from build123d import *

# Parameters (mm, degrees)
SKETCH_1_W          = 170
SKETCH_1_H          = 106
EXTRUDE_1_DEPTH     = 14
SKETCH_2_R          = 2
CUT_EXTRUDE_1_DEPTH = 5
SKETCH_3_W          = 154
SKETCH_3_H          = 87
CUT_EXTRUDE_2_DEPTH = 1


with BuildPart() as part:
    # 草图1 → 凸台-拉伸1 (new body)
    with BuildSketch(Plane.XY):
        Rectangle(SKETCH_1_W, SKETCH_1_H)
    extrude(amount=-EXTRUDE_1_DEPTH)

    # 草图2 → 切除-拉伸1 (cut)
    with BuildSketch(Plane(origin=(0, 0, -14), x_dir=(-1, 0, 0), z_dir=(0, 0, -1))):
        with Locations((37.5, 37.5)):
            Circle(SKETCH_2_R)
        with Locations((-37.5, 37.5)):
            Circle(SKETCH_2_R)
        with Locations((-37.5, -37.5)):
            Circle(SKETCH_2_R)
        with Locations((37.5, -37.5)):
            Circle(SKETCH_2_R)
    extrude(amount=-CUT_EXTRUDE_1_DEPTH, mode=Mode.SUBTRACT)

    # 草图3 → 切除-拉伸2 (cut)
    with BuildSketch(Plane.XY):
        with Locations((0, 1.5)):
            Rectangle(SKETCH_3_W, SKETCH_3_H)
    extrude(amount=-CUT_EXTRUDE_2_DEPTH, mode=Mode.SUBTRACT)


solid = part.part
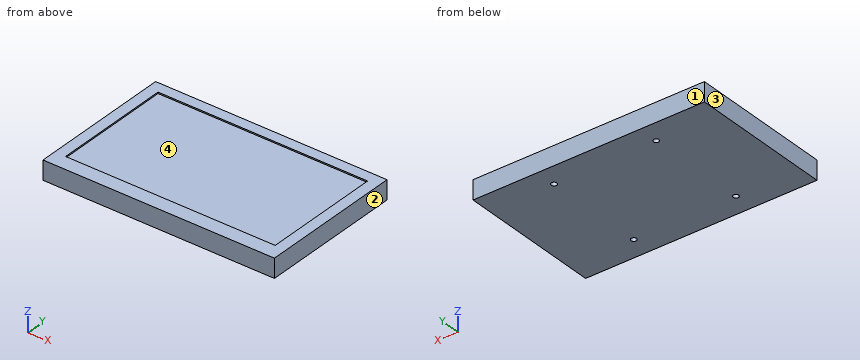
Design review of the part built by this model. Coordinates are the model's own, in mm. Face numbers are marked on the shaded views. Give positions to 0.01 mm unless a question says otherwise; leave off trailing zeros. Order: outer loops, then holes, each group sorted by start corner. A loop starts at its lowest first (then second) coordinate and runs counter-clockwise, first axis right, second up. Notation, with made-up numbers: (-8.75, -24.75) - (6.25, -24.75) arc R12 ccw to (6.25, -5.75) - close; hole circle Ø9 at (-5, 85.25). An arc over 180 degrees is marked (long way). Write item = value, one per line. Start each with the question number.
Q1. Clearance check with flat-ended pins moving along their axes: pin 1 Ø5 at (x, y) = (-37.5, 37.5) entering from +Z; pin 2 Ø2.5 at (x, y) = (37.5, 37.5) entering from -Z. State where each tip first meets the part, or that it passes through.
Q2. We need section C-C on y = -37.5. State the section outline as (x, z) points.
Q3. To check wall thickness, follow L1, parallel to Y at x = 37.5, z = -12.2; L2, parallel to Z at x = 5.5, y = -41.5. State the ranges of each line that lie inside material, in increasing order. Write a range as from..to.
Q4. We need section B-B on x = 29.5. State the section outline as (y, z) points.
Q5. Mouldability with a two-part tool opening along X and no side actions: class the marked faces 1, 2, 3 and 4 as released by +X, released by -X, zero draft, split by the parting line, or undercut.
Q6. We need section A-A on y = 32. State the section outline as (x, z) points, plus the area to 3 significant figures.
Working result:
q1.pin_1 = -1
q1.pin_2 = -9
q2.outline = (-85, -14) - (-39.5, -14) - (-39.5, -9) - (-35.5, -9) - (-35.5, -14) - (35.5, -14) - (35.5, -9) - (39.5, -9) - (39.5, -14) - (85, -14) - (85, 0) - (77, 0) - (77, -1) - (-77, -1) - (-77, 0) - (-85, 0) - close
q3.L1 = -53..-39.5, -35.5..35.5, 39.5..53
q3.L2 = -14..-1
q4.outline = (-53, -14) - (53, -14) - (53, 0) - (45, 0) - (45, -1) - (-42, -1) - (-42, 0) - (-53, 0) - close
q5.face_1 = zero draft
q5.face_2 = released by +X
q5.face_3 = released by -X
q5.face_4 = undercut
q6.outline = (-85, -14) - (85, -14) - (85, 0) - (77, 0) - (77, -1) - (-77, -1) - (-77, 0) - (-85, 0) - close
q6.area = 2,230 mm²
